Geometry check sheet. Reference: the model listing, model coordinates, mm. Face numbers are marked on the shaded views. A direction names the side the tool comes from. Round coordinates to 2 decimals unless told otherwise and drop trailing zeros. Write each loop counter-clockwise with the first axis right and the second up, starting at its lowest first coordinate (ties: lowest second). Pieces come first, ordered by that corner, then holes. Notation, with made-up numbers: M -27,55.25 L -11,55.25 A26 cw -11,88.25 Z; hole C 81,-25.5 d11. An arc over 180 degrees is marked long. Use a Markdown table: item, result.
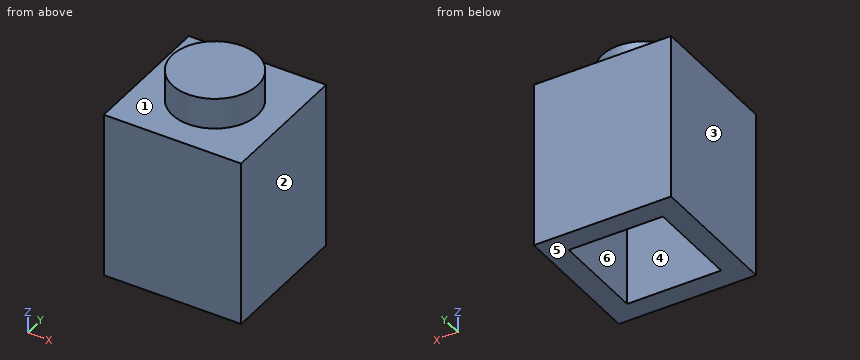
```python
from build123d import *

# Parameters (mm, degrees)
F0_W     = 7.9121
F0_H     = 7.9121
F2_DEPTH = 9.6012
F1_R     = 2.462464
F3_DEPTH = 1.778
F4_W     = 5.4229
F4_H     = 5.4229
F5_DEPTH = 7.62


with BuildPart() as f2:
    # F0 (on Top) → F2 (new body)
    with BuildSketch(Plane.XY):
        Rectangle(F0_W, F0_H)
    extrude(amount=-F2_DEPTH)

    # F1 (on face) → F3 (join)
    with BuildSketch(Plane.XY):
        Circle(F1_R)
    extrude(amount=F3_DEPTH)

    # F4 (on face) → F5 (cut)
    with BuildSketch(Plane(origin=(0, 0, -9.6012), x_dir=(1, 0, 0), z_dir=(0, 0, -1))):
        Rectangle(F4_W, F4_H)
    extrude(amount=-F5_DEPTH, mode=Mode.SUBTRACT)


solid = f2.part
```
Item 1: Go/stop test with flat-tipped pins: pin 1 (1.5 mm diameter, centred on x = -1, y = 1, fed in from -Z); pin 2 (2.5 mm diameter, centred on x = -2, y = -1.5, fed in from +Z). Record where each tip stops, or that it passes through.
Outcome:
| item | result |
|---|---|
| pin 1 | stops at z = -1.98 |
| pin 2 | stops at z = 1.78 |
Item 2: Material ranges on line 1 along Y through (x, z) = (2.25, -2.25); line 2 along Z through (x, y) = (-3.5, -0.75), recorded low to high. Write a range as from..to.
Outcome:
| item | result |
|---|---|
| line 1 | y = -3.96..-2.71, 2.71..3.96 |
| line 2 | z = -9.6..0 |
Item 3: Cross-section at A-A, the plane z = -4.25. Record the cut outline in (x, y).
Outcome:
| item | result |
|---|---|
| outline | M -3.96,-3.96 L 3.96,-3.96 L 3.96,3.96 L -3.96,3.96 Z; hole M -2.71,-2.71 L 2.71,-2.71 L 2.71,2.71 L -2.71,2.71 Z |
Item 4: Mould release check, pull along X, two halves, no side actions. Record for the marked faces 3, 4, 5 and 6: +X half, -X half, draft (parallel to the pull), parting line (faces both ways), or undercut.
Outcome:
| item | result |
|---|---|
| face 3 | -X half |
| face 4 | undercut |
| face 5 | draft |
| face 6 | undercut |
Item 5: Access from +Z, -Z, +X, -X, +Y, -Y to the whole of each face (thin tool, end or side, straight path). Record for the marked faces 1 and 2.
Outcome:
| item | result |
|---|---|
| face 1 | +Z |
| face 2 | +Z, -Z, +X, +Y, -Y |
Item 6: Cross-section at B-B, the plane y = -0.5. Record the cut outline in (x, z).
Outcome:
| item | result |
|---|---|
| outline | M -3.96,-9.6 L -2.71,-9.6 L -2.71,-1.98 L 2.71,-1.98 L 2.71,-9.6 L 3.96,-9.6 L 3.96,0 L 2.41,0 L 2.41,1.78 L -2.41,1.78 L -2.41,0 L -3.96,0 Z |
Item 7: Cross-section at D-D, the plane y = -3.25. Record the cut outline in (x, z).
Outcome:
| item | result |
|---|---|
| outline | M -3.96,-9.6 L 3.96,-9.6 L 3.96,0 L -3.96,0 Z |
